```python
from build123d import *

# Parameters (mm, degrees)
F1_DEPTH = 19.99996
F2_R     = 9.99998
F3_R     = 2.54
F4_R     = 5.10032
F5_DEPTH = 105.918


with BuildPart() as f1:
    # F0 (on Front) → F1 (new body)
    with BuildSketch(Plane.XZ):
        Polygon((14.99997, -9.99998), (112.0013, -9.99998), (112.0013, 9.99998), (14.99997, 9.99998), (14.99997, 77.99959), (-14.99997, 77.99959), (-14.99997, 9.99998), (-112.0013, 9.99998), (-112.0013, -9.99998), (-14.99997, -9.99998), (-14.99997, -77.99959), (14.99997, -77.99959), align=None)
        Polygon((74.99985, 5.50037), (74.99985, -5.50037), (7.99973, -5.50037), (7.99973, -69.99986), (-7.99973, -69.99986), (-7.99973, -5.50037), (-74.99985, -5.50037), (-74.99985, 5.50037), (-7.99973, 5.50037), (-7.99973, 69.99986), (7.99973, 69.99986), (7.99973, 5.50037), align=None, mode=Mode.SUBTRACT)
    extrude(amount=F1_DEPTH)

    # F2
    f2_edges = [f1.edges().sort_by_distance(p)[0] for p in [
        (14.99997, -9.99998, 9.99998),
        (-14.99997, -9.99998, 9.99998),
        (-14.99997, -9.99998, -9.99998),
        (14.99997, -9.99998, -9.99998),
    ]]
    fillet(f2_edges, radius=F2_R)

    # F3
    f3_edges = [f1.edges().sort_by_distance(p)[0] for p in [
        (-7.99973, -9.99998, 5.50037),
        (7.99973, -9.99998, 5.50037),
        (7.99973, -9.99998, -5.50037),
        (-7.99973, -9.99998, -5.50037),
    ]]
    fillet(f3_edges, radius=F3_R)

    # F4 (on face) → F5 (cut)
    with BuildSketch(Plane.XY.offset(9.99998)):
        with Locations((-99.90074, -10.00252)):
            Circle(F4_R)
        with Locations((99.89058, -10.00252)):
            Circle(F4_R)
    extrude(amount=-F5_DEPTH, mode=Mode.SUBTRACT)


solid = f1.part
```
Work out the finished part from the listing and answer in its coordinate system (mm). A direction names the side the tool comes from. Coordinates: 2 decimals unless noted, no trailing zeros. Loops run counter-clockwise (first coordinate to the right, second up) from the corner with the lowest first, then second, coordinate; pieces in that order, holes last.
1) Section D-D (x = 79) is taken. Give the vertices of the cut face in (y, z).
Results:
outline: (-20, -10) - (0, -10) - (0, 10) - (-20, 10) - close
2) Section B-B (x = -50.5) is taken. Give the vertices of the cut face in (y, z).
Results:
outline: (-20, -10) - (0, -10) - (0, -5.5) - (-20, -5.5) - close; (-20, 5.5) - (0, 5.5) - (0, 10) - (-20, 10) - close
3) Section A-A (z = -0.5) is taken. Give the vertices of the cut face in (x, y), plus the area to 3 significant figures.
Results:
outline: (-112, -20) - (-75, -20) - (-75, 0) - (-112, 0) - close; (75, -20) - (112, -20) - (112, 0) - (75, 0) - close; hole circle Ø10.2 at (-99.9, -10); hole circle Ø10.2 at (99.89, -10)
area: 1,320 mm2
4) For a pull along Z with two mould halves and no side action, classify faces 1 (the flat face through (-8, -10, 39)), 2 (the flat face through (-15, -10, 49)), 3 (the flat face through (0, -10, 78)) as +Z half, -Z half, draft (parallel to the pull), parting line (faces both ways), or undercut.
Results:
face 1: undercut
face 2: draft
face 3: +Z half
5) Consider probe 1 along Z at (x, y) = (61.5, -9.5); probe 2 along X at (y, z) = (-8.25, 34.5); probe 3 along X at (y, z) = (-6.25, -18.5). Determine where each line is inside the solid, lowest interval first.
Results:
probe 1: z = -10 to -5.5, 5.5 to 10
probe 2: x = -15 to -8, 8 to 15
probe 3: x = -15.11 to -8, 8 to 15.11
6) Flat-ended cylindrical pins translate along their axes: pin 1 (6 mm diameter, centred on y = -7.5, z = -43.5, fed in from +X); pin 2 (10 mm diameter, centred on y = -6, z = 14.5, fed in from -X); pin 3 (10 mm diameter, centred on x = -71.5, y = -10.5, fed in from -Z); pin 4 (4 mm diameter, centred on x = 21.5, y = -15.5, fed in from +Z). Find the tip coordinate at first contact, or state that the pin passes through.
Results:
pin 1: stops at x = 15
pin 2: stops at x = -112
pin 3: stops at z = -10
pin 4: stops at z = 11.65
7) For faces 4 (the flat face through (15, -10, -49)), 5 (the flat face through (-42, -10, -5.5)), 6 (the flat face through (-15, -10, -49)), determine the directions among +Z, -Z, +X, -X, +Y, -Y from which every point of the face is accessible in a straight line to the end or side of a thin tool.
Results:
face 4: -Z, +X, +Y, -Y
face 5: +Y, -Y
face 6: -Z, -X, +Y, -Y
8) Section C-C (z = 29) is taken. Give the vertices of the cut face in (x, y).
Results:
outline: (-15, -20) - (-8, -20) - (-8, 0) - (-15, 0) - close; (8, -20) - (15, -20) - (15, 0) - (8, 0) - close
